Can you work these out from the model? Positions are in its coordinate system, mm. A direction names the side the tool comes from. Coordinates: 2 decimals unless noted, no trailing zeros. Loops run counter-clockwise (first coordinate to the right, second up) from the corner with the lowest first, then second, coordinate; pieces in that order, holes last.
```python
from build123d import *

# Parameters (mm, degrees)
SKETCH1_R           = 0.5
BOSS_EXTRUDE1_DEPTH = 1.4
SKETCH2_R           = 2.35
CUT_EXTRUDE1_DEPTH  = 1
SKETCH3_R           = 3.5
SKETCH3_R_2         = 2.45
BOSS_EXTRUDE2_DEPTH = 2.5
SKETCH4_R           = 1.2
CUT_EXTRUDE2_DEPTH  = 20.282440198
SKETCH5_R           = 2.45
SKETCH5_R_2         = 1.2
BOSS_EXTRUDE3_DEPTH = 0.1
SKETCH6_W           = 35.735260114
SKETCH6_H           = 17.672039004
CUT_EXTRUDE4_DEPTH  = 20.513392837
CUT_EXTRUDE5_DEPTH  = 18.980545042
SCALE1_SCALE        = 0.5
SCALE2_SCALE        = 2.5


with BuildPart() as part:
    # Sketch1 → Boss-Extrude1 (new body)
    with BuildSketch(Plane(origin=(0, 0, 0), x_dir=(1, 0, 0), z_dir=(0, 1, 0))):
        with BuildLine():
            Line((-15.2, 2), (-2, 2.95))
            Line((-2, 2.95), (-2, 6.35))
            ThreePointArc((-2, 6.35), (0, 8.35), (2, 6.35))
            Line((2, 6.35), (2, 3.5))
            Line((2, 3.5), (15.2, 2))
            ThreePointArc((15.2, 2), (17.2, 0), (15.2, -2))
            Line((15.2, -2), (2, -3.5))
            Line((2, -3.5), (2, -6.35))
            ThreePointArc((2, -6.35), (0, -8.35), (-2, -6.35))
            Line((-2, -6.35), (-2, -2.95))
            Line((-2, -2.95), (-15.2, -2))
            ThreePointArc((-15.2, -2), (-17.2, 0), (-15.2, 2))
        make_face()
        with Locations((0, 6.35)):
            Circle(SKETCH1_R, mode=Mode.SUBTRACT)
        with Locations((0, 4.55)):
            Circle(SKETCH1_R, mode=Mode.SUBTRACT)
        with Locations((0, -4.55)):
            Circle(SKETCH1_R, mode=Mode.SUBTRACT)
        with Locations((0, -6.35)):
            Circle(SKETCH1_R, mode=Mode.SUBTRACT)
        with Locations((-15.2, 0)):
            Circle(SKETCH1_R, mode=Mode.SUBTRACT)
        with Locations(Location((15.2, 0, 0), (0, 0, 270))):
            Circle(SKETCH1_R, mode=Mode.SUBTRACT)
        with Locations((-13.4, 0)):
            Circle(SKETCH1_R, mode=Mode.SUBTRACT)
        with Locations((-11.6, 0)):
            Circle(SKETCH1_R, mode=Mode.SUBTRACT)
        with Locations((-9.8, 0)):
            Circle(SKETCH1_R, mode=Mode.SUBTRACT)
        with Locations((-8, 0)):
            Circle(SKETCH1_R, mode=Mode.SUBTRACT)
        with Locations((-6.2, 0)):
            Circle(SKETCH1_R, mode=Mode.SUBTRACT)
        with Locations((-4.4, 0)):
            Circle(SKETCH1_R, mode=Mode.SUBTRACT)
        with Locations(Location((13.4, 0, 0), (0, 0, 270))):
            Circle(SKETCH1_R, mode=Mode.SUBTRACT)
        with Locations(Location((11.6, 0, 0), (0, 0, 270))):
            Circle(SKETCH1_R, mode=Mode.SUBTRACT)
        with Locations(Location((9.8, 0, 0), (0, 0, 270))):
            Circle(SKETCH1_R, mode=Mode.SUBTRACT)
        with Locations(Location((8, 0, 0), (0, 0, 270))):
            Circle(SKETCH1_R, mode=Mode.SUBTRACT)
        with Locations(Location((6.2, 0, 0), (0, 0, 270))):
            Circle(SKETCH1_R, mode=Mode.SUBTRACT)
        with Locations(Location((4.4, 0, 0), (0, 0, 270))):
            Circle(SKETCH1_R, mode=Mode.SUBTRACT)
    extrude(amount=BOSS_EXTRUDE1_DEPTH)

    # Sketch2 → Cut-Extrude1 (cut)
    with BuildSketch(Plane.XZ):
        with Locations(Location((0, 0, 0), (0, 0, 270))):
            Circle(SKETCH2_R)
    extrude(amount=-CUT_EXTRUDE1_DEPTH, mode=Mode.SUBTRACT)

    # Sketch3 → Boss-Extrude2 (add)
    with BuildSketch(Plane(origin=(0, 1.4, 0), x_dir=(1, 0, 0), z_dir=(0, 1, 0))):
        with Locations(Location((0, 0, 0), (0, 0, 57.731921145))):
            Circle(SKETCH3_R)
        with Locations(Location((0, 0, 0), (0, 0, 270))):
            Circle(SKETCH3_R_2, mode=Mode.SUBTRACT)
    extrude(amount=BOSS_EXTRUDE2_DEPTH)

    # Sketch4 → Cut-Extrude2 (cut, through all)
    with BuildSketch(Plane(origin=(0, 1.4, 0), x_dir=(1, 0, 0), z_dir=(0, 1, 0))):
        with Locations(Location((0, 0, 0), (0, 0, 270))):
            Circle(SKETCH4_R)
    extrude(amount=-CUT_EXTRUDE2_DEPTH, mode=Mode.SUBTRACT)

    # Sketch5 → Boss-Extrude3 (add)
    with BuildSketch(Plane(origin=(0, 1.4, 0), x_dir=(1, 0, 0), z_dir=(0, 1, 0))):
        with Locations(Location((0, 0, 0), (0, 0, 270))):
            Circle(SKETCH5_R)
        with Locations(Location((0, 0, 0), (0, 0, 270))):
            Circle(SKETCH5_R_2, mode=Mode.SUBTRACT)
    extrude(amount=BOSS_EXTRUDE3_DEPTH)

    # Sketch6 → Cut-Extrude4 (cut, through all)
    with BuildSketch(Plane.XZ):
        Rectangle(SKETCH6_W, SKETCH6_H)
        with BuildLine():
            Line((-1.868584713, -2.959457918), (-15.2, -2))
            ThreePointArc((-15.2, -2), (-17.2, 0), (-15.2, 2))
            Line((-15.2, 2), (-1.868584713, 2.959457918))
            ThreePointArc((-1.868584713, 2.959457918), (0, 3.5), (1.868584713, 2.959457918))
            Line((1.868584713, 2.959457918), (15.2, 2))
            ThreePointArc((15.2, 2), (17.2, 0), (15.2, -2))
            Line((15.2, -2), (1.868584713, -2.959457918))
            ThreePointArc((1.868584713, -2.959457918), (0, -3.5), (-1.868584713, -2.959457918))
        make_face(mode=Mode.SUBTRACT)
    extrude(amount=-CUT_EXTRUDE4_DEPTH, mode=Mode.SUBTRACT)

    # Sketch7 → Cut-Extrude5 (cut, through all)
    with BuildSketch(Plane.XZ):
        with BuildLine():
            Line((0, 3.5), (-17.731768104, 3.5))
            Line((-17.731768104, 3.5), (-17.731768104, -3.5))
            Line((-17.731768104, -3.5), (0, -3.5))
            ThreePointArc((0, -3.5), (-3.5, 0), (0, 3.5))
        make_face()
    extrude(amount=-CUT_EXTRUDE5_DEPTH, mode=Mode.SUBTRACT)


with BuildPart() as part_1:
    # Scale1: scaled about (4.675225988, 1.286509447, 0)
    add(part.part.scale(SCALE1_SCALE).moved(Location((2.337612994, 0.643254724, 0))))


with BuildPart() as part_2:
    # Scale2: scaled about (4.675225988, 1.286509447, 0)
    add(part_1.part.scale(SCALE2_SCALE).moved(Location((-7.012838982, -1.92976417, 0))))


solid = part_2.part
```
(1) Which directions (+Z, -Z, +X, -X, +Y, -Y) give clear straight access to the entire face, cutting with the end or side of a thin tool? Please do faces 5 (the cylindrical face through (3.721, 0.541, -0.135)), 6 (the cylindrical face through (-2.96, 0.29, 2.33)), 7 (the cylindrical face through (-0.25, 3.03, 2.92)).
Check values:
face 5: +Y, -Y
face 6: -Y
face 7: +Y
(2) I'm going to push flat-ended pins straight in: pin 1 (2 mm diameter, centred on x = 15.58, z = 0, fed in from -Y); pin 2 (3.5 mm diameter, centred on x = -1.17, z = 0, fed in from +Y). Where does each tip first touch, or does it pass through?
Check values:
pin 1: stops at y = -0.32
pin 2: stops at y = 1.55
(3) If we mould it in two halves opening along X, with no side actions, what happens to faces 1 (the cylindrical face through (16.2, 0.5, -0.1)), 2 (the cylindrical face through (13.95, 0.54, -0.08)), 3 (the flat face through (-4, 4.553, 2)), 4 (the cylindrical face through (20.33, 0.54, -0.05))? For each: released by +X, released by -X, zero draft, split by the parting line, or undercut.
Check values:
face 1: undercut
face 2: undercut
face 3: zero draft
face 4: released by +X
(4) I want a section at D-D on z = 0. State how many separate pieces and enclosed holes the cut face has, then the cut area to 3 significant figures.
Check values:
separate pieces: 9
enclosed holes: 0
area: 29.7 mm2
(5) I want a section at B-B on x = 15.25. Write out the boundary of the cut face in (y, z), then the cut area to 3 significant figures.
Check values:
outline: (-0.32, -2.69) - (1.43, -2.69) - (1.43, -0.53) - (-0.32, -0.53) - close; (-0.32, 0.53) - (1.43, 0.53) - (1.43, 2.69) - (-0.32, 2.69) - close
area: 7.55 mm2
(6) I want a section at A-A on z = -1. Write out the boundary of the cut face in (x, y), then the cut area to 3 significant figures.
Check values:
outline: (-5.43, -0.32) - (-3.93, -0.32) - (-3.93, 0.93) - (-2.29, 0.93) - (-2.29, 1.55) - (-4.06, 1.55) - (-4.06, 4.55) - (-5.43, 4.55) - close; (-0.05, 0.93) - (1.59, 0.93) - (1.59, -0.32) - (20.12, -0.32) - (20.12, 1.43) - (3.09, 1.43) - (3.09, 4.55) - (1.73, 4.55) - (1.73, 1.55) - (-0.05, 1.55) - close
area: 45.7 mm2
(7) If I drill on probe 1 along X at (y, z) = (1.6, 0); probe 2 along X at (y, z) = (1.5, 0); probe 3 along Y at (x, z) = (1.75, -3.5), over which ranges is the centre line in solid material (lowest first)?
Check values:
probe 1: x = -5.54 to -4.23, 1.89 to 3.21
probe 2: x = -5.54 to -2.67, 0.33 to 3.21
probe 3: y = -0.32 to 1.43
